from build123d import *

# Parameters (mm, degrees)
SKETCH1_R           = 52
BOSS_EXTRUDE1_DEPTH = 140
SHELL1_T            = 8
CUT_EXTRUDE1_START  = -40
SKETCH3_R           = 44
CUT_EXTRUDE1_DEPTH  = 40


with BuildPart() as part:
    # Sketch1 → Boss-Extrude1 (new body)
    with BuildSketch(Plane(origin=(0, 0, 0), x_dir=(1, 0, 0), z_dir=(0, 1, 0))):
        with Locations(Location((0, 0, 0), (0, 0, 270))):
            Circle(SKETCH1_R)
    extrude(amount=BOSS_EXTRUDE1_DEPTH)

    # Shell1 (no face opened: a closed hollow body)
    add(offset(amount=-SHELL1_T, mode=Mode.PRIVATE), mode=Mode.SUBTRACT)

    # Sketch3 → Cut-Extrude1 (cut)
    with BuildSketch(Plane(origin=(0, 140, 0), x_dir=(1, 0, 0), z_dir=(0, 1, 0)).offset(CUT_EXTRUDE1_START)):
        with Locations(Location((0, 0, 0), (0, 0, 270))):
            Circle(SKETCH3_R)
    extrude(amount=CUT_EXTRUDE1_DEPTH, mode=Mode.SUBTRACT)


solid = part.part
Geometry: final body of the model. Coordinates: model frame, mm. A direction names the side the tool comes from. Round coordinates to 2 decimals unless told otherwise and drop trailing zeros. Order: outer loops, then holes, each group sorted by start corner. A loop starts at its lowest first (then second) coordinate and runs counter-clockwise, first axis right, second up. Notation, with made-up numbers: (58, 23) -> (79, 23) arc R9 cw to (79, 31) -> close; hole circle Ø8 at (-15, -3.75). An arc over 180 degrees is marked (long way). Put each result on its own line as item: value. Start each with the question number.
Q1. Section A-A on x = 0. Return the cut outline in (y, z), and give its area (3 significant figures).
Q2. Reachability of faces 1 (the flat face through (1, 8, -1)), 2 (the flat face through (1, 0, -1)) from +Z, -Z, +X, -X, +Y, -Y: full face, straight path, thin tool, end or side. Return the list, or none.
Q3. Section B-B on z = 0. Return the cut outline in (x, y).
Q4. First-contact query: pin 1 (8 mm diameter, centred on x = 30.5, z = -4, fed in from +Y); pin 2 (8 mm diameter, centred on y = 18, z = 21, fed in from +X); pin 3 (10 mm diameter, centred on x = 16, y = 19.5, fed in from -Z). Flat tips, straight axial feed; report the tip coordinate or a pass-through.
Q5. Pull-direction query (Z, two-part tool) for faces 3 (the flat face through (12, 140, -43)), 4 (the cylindrical face through (-31.641, 69.02, -41.265)), 5 (the cylindrical face through (-42.954, 73.076, -9.538)); classes: +Z half, -Z half, draft (parallel to the pull), parting line (faces both ways), or undercut.
Q6. Line query: probe 1 along X at (y, z) = (58.5, 0); probe 2 along Y at (x, z) = (-8.5, 15.5); probe 3 along Z at (x, y) = (31, 64). Output: solid intervals per line, ascending.
Q7. Section C-C on y = 62. Return the cut outline in (x, z).
Ans:
1. outline: (0, -52) -> (140, -52) -> (140, -44) -> (8, -44) -> (8, 44) -> (140, 44) -> (140, 52) -> (0, 52) -> close
1. area: 2,940 mm2
2. face 1: +Y
2. face 2: +Z, -Z, +X, -X, -Y
3. outline: (-52, 0) -> (52, 0) -> (52, 140) -> (44, 140) -> (44, 8) -> (-44, 8) -> (-44, 140) -> (-52, 140) -> close
4. pin 1: stops at y = 8
4. pin 2: stops at x = 49.14
4. pin 3: stops at z = -50.82
5. face 3: draft
5. face 4: parting line
5. face 5: undercut
6. probe 1: x = -52 to -44, 44 to 52
6. probe 2: y = 0 to 8
6. probe 3: z = -41.75 to -31.22, 31.22 to 41.75
7. outline: circle Ø104 at (0, 0); hole circle Ø88 at (0, 0)
